from build123d import *

# Parameters (mm, degrees)
SKIZZE1_W                       = 50
SKIZZE1_H                       = 185
AUFSATZ_LINEAR_AUSTRAGEN1_DEPTH = 10
SKIZZE3_W                       = 10
SKIZZE3_H                       = 10
AUFSATZ_LINEAR_AUSTRAGEN3_DEPTH = 50
SKIZZE4_R                       = 2
SCHNITT_LINEAR_AUSTRAGEN1_DEPTH = 97.33924434
SKIZZE6_W                       = 50
SKIZZE6_H                       = 50
AUFSATZ_LINEAR_AUSTRAGEN4_DEPTH = 10
SKIZZE7_R                       = 1
SCHNITT_LINEAR_AUSTRAGEN2_DEPTH = 125.524094054
SKIZZE8_R                       = 1
SCHNITT_LINEAR_AUSTRAGEN3_DEPTH = 10


with BuildPart() as part:
    # Skizze1 → Aufsatz-Linear austragen1 (new body)
    with BuildSketch(Plane(origin=(0, 0, 0), x_dir=(0, 0, -1), z_dir=(1, 0, 0))):
        Rectangle(SKIZZE1_W, SKIZZE1_H)
    extrude(amount=AUFSATZ_LINEAR_AUSTRAGEN1_DEPTH)

    # Skizze3 → Aufsatz-Linear austragen3 (add)
    with BuildSketch(Plane.XY.offset(25)):
        with Locations((15, 47.5)):
            Rectangle(SKIZZE3_W, SKIZZE3_H)
        with Locations((15, -7.5)):
            Rectangle(SKIZZE3_W, SKIZZE3_H)
    extrude(amount=-AUFSATZ_LINEAR_AUSTRAGEN3_DEPTH)

    # Skizze4 → Schnitt-Linear austragen1 (cut, through all)
    with BuildSketch(Plane(origin=(10, 0, 0), x_dir=(0, 0, -1), z_dir=(1, 0, 0))):
        with Locations((0, -72.5)):
            Circle(SKIZZE4_R)
    extrude(amount=-SCHNITT_LINEAR_AUSTRAGEN1_DEPTH, mode=Mode.SUBTRACT)

    # Skizze6 → Aufsatz-Linear austragen4 (add)
    with BuildSketch(Plane(origin=(0, 92.5, 0), x_dir=(1, 0, 0), z_dir=(0, 1, 0))):
        with Locations((25, 0)):
            Rectangle(SKIZZE6_W, SKIZZE6_H)
    extrude(amount=AUFSATZ_LINEAR_AUSTRAGEN4_DEPTH)

    # Skizze7 → Schnitt-Linear austragen2 (cut, through all)
    with BuildSketch(Plane.XY.offset(25)):
        with Locations((5, 80)):
            Circle(SKIZZE7_R)
        with Locations((5, 55)):
            Circle(SKIZZE7_R)
    extrude(amount=-SCHNITT_LINEAR_AUSTRAGEN2_DEPTH, mode=Mode.SUBTRACT)

    # Skizze8 → Schnitt-Linear austragen3 (cut)
    with BuildSketch(Plane(origin=(50, 0, 0), x_dir=(0, 0, -1), z_dir=(1, 0, 0))):
        with Locations((-15, 97.5)):
            Circle(SKIZZE8_R)
        with Locations((15, 97.5)):
            Circle(SKIZZE8_R)
    extrude(amount=-SCHNITT_LINEAR_AUSTRAGEN3_DEPTH, mode=Mode.SUBTRACT)


solid = part.part
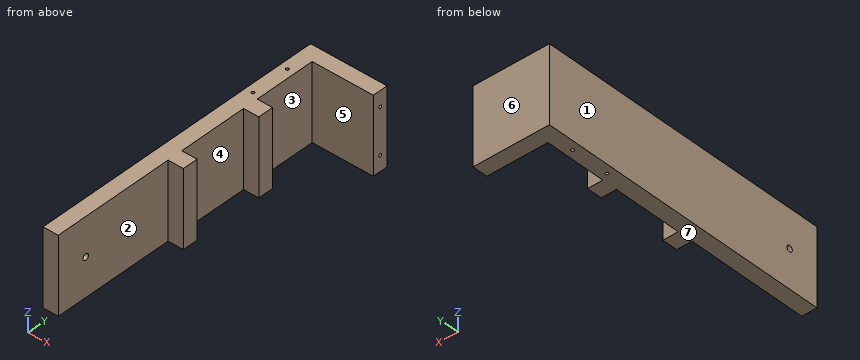
Design review of the part built by this model. Coordinates are the model's own, in mm. Face numbers are marked on the shaded views. A direction names the side the tool comes from. Give positions to 0.01 mm unless a question says otherwise; leave off trailing zeros. Order: outer loops, then holes, each group sorted by start corner. A loop starts at its lowest first (then second) coordinate and runs counter-clockwise, first axis right, second up. Notation, with made-up numbers: (-4, 50) - (25, 50) arc R21 cw to (25, 80) - close; hole circle Ø3 at (-21.75, -33.75). An arc over 180 degrees is marked (long way). Use CSV: the item, a comma, the result in double quotes. Start each with the question number.
Q1. For P1, Ø3, axis at x = 14, z = -8, coming from the -Y side; P2, Ø12, axis at y = 69, z = -3, coming from the +X side; P3, Ø1.2, axis at x = 5, y = 55, coming from the -Z side; P4, Ø5, axis at y = -9, z = 11.5, coming from the +X side, all flat-tipped, find the tip position at first contact; note any pin that passes through.
Q2. Draft analysis for pull direction Y (two halves, no side actions). For the marked faces 4, 5, 6 and 7, state which applies: pulls with the +Y half, pulls with the -Y half, needs draft (parallel to the pull), parting line crosses it, or undercut.
Q3. For line 1 (Z direction, x = 42.25, y = 97.5); line 2 (Y direction, x = 5.25, z = 0); line 3 (Y direction, x = 18.5, z = -15.5), list the stretches that pass through material, from the lowest coordinate up.
Q4. Take a section at D-D (x = 44). State the section outline as (y, z) points.
Q5. Take a section at B-B (z = 0). State the section outline as (x, y) points.
Q6. Machinability: for the marked faces 1, 2 and 3, which of the approach directions +Z, -Z, +X, -X, +Y, -Y give a long, thin tool a straight path to every point of the face, cutting with its end or side? Answer none if there is none.
Q7. Take a section at C-C (z = -8). State the section outline as (x, y) points.
Q8. Take a section at A-A (y = -72.5). State the section outline as (x, z) points, and give its area (3 significant figures).
Calculated:
1,P1,"stops at y = -12.5"
1,P2,"stops at x = 10"
1,P3,"passes through"
1,P4,"stops at x = 20"
2,face 4,"undercut"
2,face 5,"undercut"
2,face 6,"pulls with the +Y half"
2,face 7,"needs draft"
3,line 1,"z = -25 to -16, -14 to 14, 16 to 25"
3,line 2,"y = -92.5 to -74.5, -70.5 to 54.03, 55.97 to 79.03, 80.97 to 102.5"
3,line 3,"y = -12.5 to -2.5, 42.5 to 52.5, 92.5 to 102.5"
4,outline,"(92.5, -25) - (102.5, -25) - (102.5, 25) - (92.5, 25) - close; hole circle Ø2 at (97.5, -15); hole circle Ø2 at (97.5, 15)"
5,outline,"(0, -92.5) - (10, -92.5) - (10, -74.5) - (0, -74.5) - close; (0, -70.5) - (10, -70.5) - (10, -12.5) - (20, -12.5) - (20, -2.5) - (10, -2.5) - (10, 42.5) - (20, 42.5) - (20, 52.5) - (10, 52.5) - (10, 92.5) - (50, 92.5) - (50, 102.5) - (0, 102.5) - close; hole circle Ø2 at (5, 55); hole circle Ø2 at (5, 80)"
6,face 1,"+Z, -Z, -X, +Y, -Y"
6,face 2,"+Z, -Z, +X, -Y"
6,face 3,"+Z, -Z, +X"
7,outline,"(0, -92.5) - (10, -92.5) - (10, -12.5) - (20, -12.5) - (20, -2.5) - (10, -2.5) - (10, 42.5) - (20, 42.5) - (20, 52.5) - (10, 52.5) - (10, 92.5) - (50, 92.5) - (50, 102.5) - (0, 102.5) - close; hole circle Ø2 at (5, 55); hole circle Ø2 at (5, 80)"
8,outline,"(0, -25) - (10, -25) - (10, -2) - (0, -2) - close; (0, 2) - (10, 2) - (10, 25) - (0, 25) - close"
8,area,"460 mm²"
